Source: CAD feature listing. Evaluate the final solid. Frame: model axes, mm. A direction names the side the tool comes from. Round coordinates to 2 decimals unless told otherwise and drop trailing zeros.
from build123d import *

# Parameters (mm, degrees)
ESQUISSE1_W             = 40
ESQUISSE1_H             = 35
ESQUISSE1_W_2           = 12
ESQUISSE1_H_2           = 2.5
BOSS_EXTRU_1_DEPTH      = 2
ENL_V_MAT_EXTRU_1_DEPTH = 10


with BuildPart() as part:
    # Esquisse1 → Boss.-Extru.1 (new body)
    with BuildSketch(Plane.XY):
        Rectangle(ESQUISSE1_W, ESQUISSE1_H)
        with Locations((-9, -11.25)):
            Rectangle(ESQUISSE1_W_2, ESQUISSE1_H_2, mode=Mode.SUBTRACT)
    extrude(amount=BOSS_EXTRU_1_DEPTH)

    # Esquisse2 → Enlèv. mat.-Extru.1 (cut)
    with BuildSketch(Plane.XY.offset(2)):
        with BuildLine():
            Line((-28.997409478, -17.623933779), (-30.265364491, 23.868234326))
            Line((-30.265364491, 23.868234326), (4.12, 17.5))
            add(Edge.make_bspline(
                [(4.12, 17.5), (-20.235504114, 6.589370836), (-28.997409478, -17.623933779)],
                knots=[0, 0, 0, 1, 1, 1], degree=2))
        make_face()
    extrude(amount=-ENL_V_MAT_EXTRU_1_DEPTH, mode=Mode.SUBTRACT)


solid = part.part
1) Reachability of faces 5 (the face through (4, 0, 2)), 6 (the face through (-15, -11, 1)) from +Z, -Z, +X, -X, +Y, -Y: full face, straight path, thin tool, end or side. Return the list, or none.
Taken from the geometry:
face 5: +Z, +X, -X, +Y, -Y
face 6: +Z, -Z
2) Pull-direction query (X, two-part tool) for faces 1 (the face through (-9, -12.5, 1)), 2 (the face through (20, 0, 1)), 3 (the face through (4, 0, 0)), 4 (the face through (-20, -9, 1)); classes: released by +X, released by -X, zero draft, split by the parting line, or undercut.
Taken from the geometry:
face 1: undercut
face 2: released by +X
face 3: zero draft
face 4: released by -X
3) Material intervals for line 1 (X direction, y = -12, z = 1.4); line 2 (Y direction, x = -11, z = 0.4); line 3 (X direction, y = 15.5, z = 0.9), sorted ascending.
Taken from the geometry:
line 1: x = -20 to -15, -3 to 20
line 2: y = -17.5 to -12.5, -10 to 8.25
line 3: x = 0 to 20
4) Contact query for a flat-ended pin moving along its axis: P1, Ø1, axis at x = -10, z = 1, coming from the +Y side. Output: stop coordinate, or through.
Taken from the geometry:
P1: stops at y = 9.44
